Part model, mm, in its own coordinate system. Face numbers are marked on the shaded views. Round coordinates to 2 decimals unless told otherwise and drop trailing zeros. Loops run counter-clockwise (first coordinate to the right, second up) from the corner with the lowest first, then second, coordinate; pieces in that order, holes last. Notation, with made-up numbers: M 5,27.5 L 45,27.5 A18 ccw 45,54.5 Z; hole C 70.5,85 d7. An arc over 180 degrees is marked long. Put each result on its own line as item: value. Start each with the question number.
1) Probe line 1 along Y through (x, z) = (-36, 1.6); line 2 along X through (y, z) = (8, 1.1); line 3 along X through (y, z) = (6.75, 0.6). List the from-to ranges inside material, lowest first.
2) Pull direction X, two halves, no side cores. Call the marked faces 1 and 2: +X half, -X half, draft (parallel to the pull), parting line (faces both ways), or undercut.
3) Drop flat-ended pins along their axis: pin 1 Ø0.6 at (x, z) = (-37.5, 1.5) entering from +Y; pin 2 Ø1.2 at (x, y) = (-34.09, 7.88) entering from +Z; pin 3 Ø1 at (y, z) = (-9.5, 0.5) entering from -X. Give the stop position or say it passes through.
4) Slice it at C-C on x = -16.5. Give the cut face in (y, z), then the cut area to 3 significant figures.
5) Slice it at D-D on z = 0.3. Give the cut face in (x, y), then the cut area to 3 significant figures.
6) Slice it at B-B on y = 8.5. Give the cut face in (x, z).
7) Slice it at A-A on x = -34. Give the cut face in (y, z).
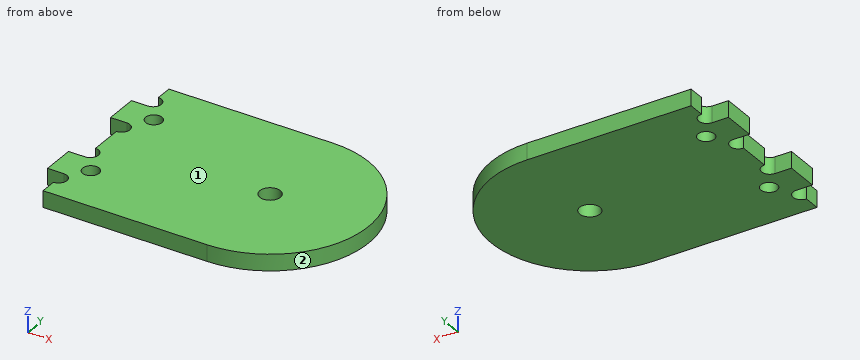
```python
from build123d import *

# Parameters (mm, degrees)
SKETCH_1_R      = 1.25
SKETCH_1_R_2    = 1
EXTRUDE_1_DEPTH = 2


with BuildPart() as part:
    # 草圖1 → 填料-伸長1 (new body)
    with BuildSketch(Plane.XY):
        with BuildLine():
            Line((-36.093061493, 13.879025542), (-16.093061493, 13.879025542))
            ThreePointArc((-16.093061493, 13.879025542), (-4.093061493, 1.879025542), (-16.093061493, -10.120974458))
            Line((-16.093061493, -10.120974458), (-36.093061493, -10.120974458))
            Line((-36.093061493, -10.120974458), (-36.093061493, -8.120974458))
            ThreePointArc((-36.093061493, -8.120974458), (-35.093061493, -7.120974458), (-36.093061493, -6.120974458))
            Line((-36.093061493, -6.120974458), (-38.093061493, -6.120974458))
            Line((-38.093061493, -6.120974458), (-38.093061493, -2.120974458))
            Line((-38.093061493, -2.120974458), (-36.093061493, -2.120974458))
            ThreePointArc((-36.093061493, -2.120974458), (-35.093061493, -1.120974458), (-36.093061493, -0.120974458))
            Line((-36.093061493, -0.120974458), (-36.093061493, 3.879025542))
            ThreePointArc((-36.093061493, 3.879025542), (-35.093061493, 4.879025542), (-36.093061493, 5.879025542))
            Line((-36.093061493, 5.879025542), (-38.093061493, 5.879025542))
            Line((-38.093061493, 5.879025542), (-38.093061493, 9.879025542))
            Line((-38.093061493, 9.879025542), (-36.093061493, 9.879025542))
            ThreePointArc((-36.093061493, 9.879025542), (-35.093061493, 10.879025542), (-36.093061493, 11.879025542))
            Line((-36.093061493, 11.879025542), (-36.093061493, 13.879025542))
        make_face()
        with Locations((-16.093061493, 1.879025542)):
            Circle(SKETCH_1_R, mode=Mode.SUBTRACT)
        with Locations((-34.093061493, 7.879025542)):
            Circle(SKETCH_1_R_2, mode=Mode.SUBTRACT)
        with Locations((-34.093061493, -4.120974458)):
            Circle(SKETCH_1_R_2, mode=Mode.SUBTRACT)
    extrude(amount=EXTRUDE_1_DEPTH)


solid = part.part
```
Recorded:
1. line 1: y = -10.12 to -8.12, -6.13 to -2.12, -0.13 to 3.88, 5.87 to 9.88, 11.87 to 13.88
1. line 2: x = -38.09 to -35.09, -33.1 to -5.77
1. line 3: x = -38.09 to -5.13
2. face 1: draft
2. face 2: +X half
3. pin 1: stops at y = 9.88
3. pin 2: passes through
3. pin 3: stops at x = -36.09
4. outline: M -10.12,0 L 0.7,0 L 0.7,2 L -10.12,2 Z; M 3.06,0 L 13.88,0 L 13.88,2 L 3.06,2 Z
4. area: 43.3 mm2
5. outline: M -38.09,-6.12 L -36.09,-6.12 A1 cw -36.09,-8.12 L -36.09,-10.12 L -16.09,-10.12 A12 ccw -16.09,13.88 L -36.09,13.88 L -36.09,11.88 A1 cw -36.09,9.88 L -38.09,9.88 L -38.09,5.88 L -36.09,5.88 A1 cw -36.09,3.88 L -36.09,-0.12 A1 cw -36.09,-2.12 L -38.09,-2.12 Z; hole C -34.09,-4.12 d2; hole C -34.09,7.88 d2; hole C -16.09,1.88 d2.5
5. area: 705 mm2
6. outline: M -38.09,0 L -34.88,0 L -34.88,2 L -38.09,2 Z; M -33.31,0 L -6.08,0 L -6.08,2 L -33.31,2 Z
7. outline: M -10.12,0 L -5.12,0 L -5.12,2 L -10.12,2 Z; M -3.13,0 L 6.88,0 L 6.88,2 L -3.13,2 Z; M 8.87,0 L 13.88,0 L 13.88,2 L 8.87,2 Z
